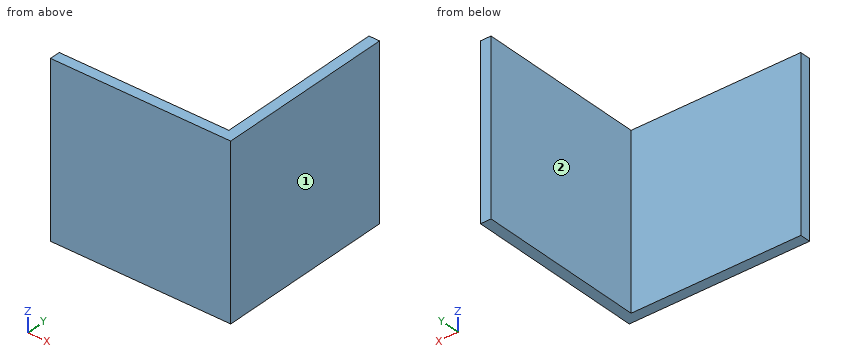
Autodesk Inventor part; units mm, degrees
ref_plane "YZ Plane" through (0, 0, 0) normal (1, 0, 0) x (0, 1, 0)
ref_plane "XZ Plane" through (0, 0, 0) normal (0, 1, 0) x (-1, 0, 0)
ref_plane "XY Plane" through (0, 0, 0) normal (0, 0, 1) x (1, 0, 0)
sketch "Sketch1" plane through (0, 0, 0) normal (0, 1, 0) x (-1, 0, 0)
  line L0 (0, 0) -> (53.975, 0)
  line L1 (53.975, 0) -> (53.975, -50.8)
  line L2 (53.975, -50.8) -> (0, -50.8)
  line L3 (0, -50.8) -> (0, 0)
  dimension "d0" = 53.975
  dimension "d1" = 50.8
extrude "Extrusion1" add sketch "Sketch1" along normal blind 3.175
sketch "Sketch2" plane through (0, 3.175, 0) normal (0, 1, 0) x (1, 0, 0)
  line L0 (0, 50.8) -> (-53.975, 50.8)
  line L1 (0, 0) -> (-3.175, 0)
  line L2 (-3.175, 0) -> (-3.175, 50.8)
  line L3 (-3.175, 50.8) -> (0, 50.8)
  line L4 (0, 50.8) -> (0, 0)
  dimension "d4" = 3.175
extrude "Extrusion2" add sketch "Sketch2" along normal blind 50.8
properties part number "H"
Geometry check sheet. Reference: the model listing, model coordinates, mm. Face numbers are marked on the shaded views. A direction names the side the tool comes from. Give positions to 0.01 mm unless a question says otherwise; leave off trailing zeros. Order: outer loops, then holes, each group sorted by start corner. A loop starts at its lowest first (then second) coordinate and runs counter-clockwise, first axis right, second up.
1) Cross-section at B-B (y = 36.5). Record the boundary of the cut face in (x, z) (3 decimals), then the cut area to 3 significant figures.
Results are:
outline: (-3.175, -50.8) - (0, -50.8) - (0, 0) - (-3.175, 0) - close
area: 161 mm2
2) Tool access check on the marked faces 1 and 2. Record the directions out of +Z, -Z, +X, -X, +Y, -Y that give a thin tool (end or side, any length) a straight path to the whole face; none if there is none.
Results are:
face 1: +Z, -Z, +X, +Y, -Y
face 2: +Z, -Z, -X, +Y
3) Cross-section at C-C (x = -48). Record the boundary of the cut face in (y, z) (3 decimals), then the cut area to 3 significant figures.
Results are:
outline: (0, -50.8) - (3.175, -50.8) - (3.175, 0) - (0, 0) - close
area: 161 mm2
4) Gauge pin test, flat ends, axial feed: pin 1 (1 mm diameter, centred on y = 40, z = -45.5, fed in from -X) (3 decimals); pin 2 (3 mm diameter, centred on y = 5.5, z = -28.5, fed in from +X). Record the tip position at first contact, or that the pin passes through.
Results are:
pin 1: stops at x = -3.175
pin 2: stops at x = 0
5) Cross-section at A-A (z = -47). Record the boundary of the cut face in (x, y) (3 decimals), then the cut area to 3 significant figures.
Results are:
outline: (-53.975, 0) - (0, 0) - (0, 53.975) - (-3.175, 53.975) - (-3.175, 3.175) - (-53.975, 3.175) - close
area: 333 mm2
6) Material ranges on probe 1 along X at (y, z) = (22, -47.5) (3 decimals); probe 2 along Y at (x, z) = (-22.5, -16) (3 decimals), recorded low to high.
Results are:
probe 1: x = -3.175 to 0
probe 2: y = 0 to 3.175
